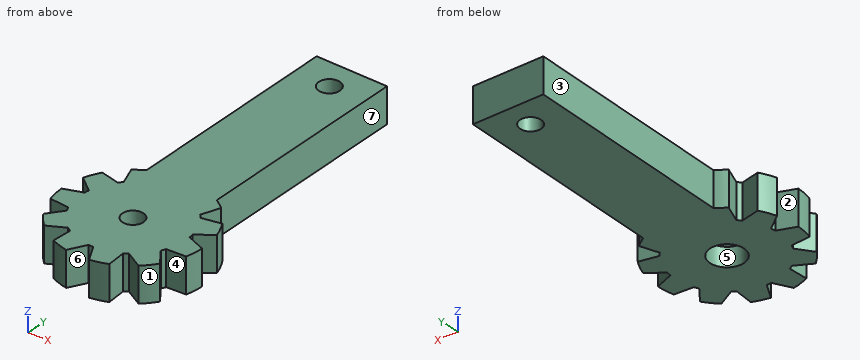
from build123d import *

# Parameters (mm, degrees)
BOSS_EXTRUDE1_DEPTH = 5
SKETCH5_R           = 2.425
CUT_EXTRUDE2_DEPTH  = 2.7
SKETCH6_R           = 1.5
CUT_EXTRUDE3_DEPTH  = 12
SKETCH7_W           = 10
SKETCH7_H           = 35
BOSS_EXTRUDE3_DEPTH = 5
SKETCH8_R           = 1.5
CUT_EXTRUDE4_DEPTH  = 12


with BuildPart() as part:
    # Sketch1 → Boss-Extrude1 (new body)
    with BuildSketch(Plane.XY):
        with BuildLine():
            Line((-1.212917817, 9.926168967), (-1.792316692, 7.28269187))
            ThreePointArc((-1.792316692, 7.28269187), (-2.112994176, 7.196197302), (-2.429527737, 7.095589826))
            Line((-2.429527737, 7.095589826), (-4.346120706, 9.006177592))
            ThreePointArc((-4.346120706, 9.006177592), (-5.406408175, 8.412535328), (-6.386863504, 7.694671831))
            Line((-6.386863504, 7.694671831), (-5.445113235, 5.157590703))
            ThreePointArc((-5.445113235, 5.157590703), (-5.668121808, 4.911455505), (-5.880014276, 4.655688147))
            Line((-5.880014276, 4.655688147), (-8.525296613, 5.226788465))
            ThreePointArc((-8.525296613, 5.226788465), (-9.096319954, 4.15415013), (-9.533025155, 3.020170756))
            Line((-9.533025155, 3.020170756), (-7.369124799, 1.394990929))
            ThreePointArc((-7.369124799, 1.394990929), (-7.423660814, 1.067361287), (-7.463637828, 0.737638377))
            Line((-7.463637828, 0.737638377), (-9.997751083, -0.212069068))
            ThreePointArc((-9.997751083, -0.212069068), (-9.898214419, -1.423148383), (-9.652518677, -2.613213194))
            Line((-9.652518677, -2.613213194), (-6.953491308, -2.810508608))
            ThreePointArc((-6.953491308, -2.810508608), (-6.822239965, -3.115612598), (-6.677609105, -3.414606366))
            Line((-6.677609105, -3.414606366), (-8.295990224, -5.583596171))
            ThreePointArc((-8.295990224, -5.583596171), (-7.557495744, -6.548607339), (-6.70740572, -7.416920419))
            Line((-6.70740572, -7.416920419), (-4.330173457, -6.12369152))
            ThreePointArc((-4.330173457, -6.12369152), (-4.054806131, -6.309401496), (-3.771486674, -6.482737714))
            Line((-3.771486674, -6.482737714), (-3.960311086, -9.182370941))
            ThreePointArc((-3.960311086, -9.182370941), (-2.817325568, -9.594929736), (-1.63273884, -9.865807817))
            Line((-1.63273884, -9.865807817), (-0.332056129, -7.492645643))
            ThreePointArc((-0.332056129, -7.492645643), (0, -7.5), (0.332056129, -7.492645643))
            Line((0.332056129, -7.492645643), (1.63273884, -9.865807817))
            ThreePointArc((1.63273884, -9.865807817), (2.817325568, -9.594929736), (3.960311086, -9.182370941))
            Line((3.960311086, -9.182370941), (3.771486674, -6.482737714))
            ThreePointArc((3.771486674, -6.482737714), (4.054806131, -6.309401496), (4.330173457, -6.12369152))
            Line((4.330173457, -6.12369152), (6.70740572, -7.416920419))
            ThreePointArc((6.70740572, -7.416920419), (7.557495744, -6.548607339), (8.295990224, -5.583596171))
            Line((8.295990224, -5.583596171), (6.677609105, -3.414606366))
            ThreePointArc((6.677609105, -3.414606366), (6.822239965, -3.115612598), (6.953491308, -2.810508608))
            Line((6.953491308, -2.810508608), (9.652518677, -2.613213194))
            ThreePointArc((9.652518677, -2.613213194), (9.898214419, -1.423148383), (9.997751083, -0.212069068))
            Line((9.997751083, -0.212069068), (7.463637828, 0.737638377))
            ThreePointArc((7.463637828, 0.737638377), (7.423660814, 1.067361287), (7.369124799, 1.394990929))
            Line((7.369124799, 1.394990929), (9.533025155, 3.020170756))
            ThreePointArc((9.533025155, 3.020170756), (9.096319954, 4.15415013), (8.525296613, 5.226788465))
            Line((8.525296613, 5.226788465), (5.880014276, 4.655688147))
            ThreePointArc((5.880014276, 4.655688147), (5.668121808, 4.911455505), (5.445113235, 5.157590703))
            Line((5.445113235, 5.157590703), (6.386863504, 7.694671831))
            ThreePointArc((6.386863504, 7.694671831), (5.406408175, 8.412535328), (4.346120706, 9.006177592))
            Line((4.346120706, 9.006177592), (2.429527737, 7.095589826))
            ThreePointArc((2.429527737, 7.095589826), (2.112994176, 7.196197302), (1.792316692, 7.28269187))
            Line((1.792316692, 7.28269187), (1.212917817, 9.926168967))
            ThreePointArc((1.212917817, 9.926168967), (0, 10), (-1.212917817, 9.926168967))
        make_face()
    extrude(amount=BOSS_EXTRUDE1_DEPTH)

    # Sketch5 → Cut-Extrude2 (cut)
    with BuildSketch(Plane(origin=(0, 0, 0), x_dir=(-1, 0, 0), z_dir=(0, 0, -1))):
        Circle(SKETCH5_R)
    extrude(amount=-CUT_EXTRUDE2_DEPTH, mode=Mode.SUBTRACT)

    # Sketch6 → Cut-Extrude3 (cut)
    with BuildSketch(Plane(origin=(0, 0, 2.7), x_dir=(-1, 0, 0), z_dir=(0, 0, -1))):
        Circle(SKETCH6_R)
    extrude(amount=-CUT_EXTRUDE3_DEPTH, mode=Mode.SUBTRACT)

    # Sketch7 → Boss-Extrude3 (add)
    with BuildSketch(Plane(origin=(0, 0, 0), x_dir=(-1, 0, 0), z_dir=(0, 0, -1))):
        with Locations((0, 21.5)):
            Rectangle(SKETCH7_W, SKETCH7_H)
    extrude(amount=-BOSS_EXTRUDE3_DEPTH)

    # Sketch8 → Cut-Extrude4 (cut)
    with BuildSketch(Plane(origin=(0, 0, 0), x_dir=(-1, 0, 0), z_dir=(0, 0, -1))):
        with Locations((0, 35)):
            Circle(SKETCH8_R)
    extrude(amount=-CUT_EXTRUDE4_DEPTH, mode=Mode.SUBTRACT)


solid = part.part
Build history of the part. All positions in model axes, mm. Face numbers are marked on the shaded views. A direction names the side the tool comes from. Give positions to 0.01 mm unless a question says otherwise; leave off trailing zeros. Order: outer loops, then holes, each group sorted by start corner. A loop starts at its lowest first (then second) coordinate and runs counter-clockwise, first axis right, second up. Notation, with made-up numbers: M 28,-5 L 83,-5 A30 cw 83,24 Z; hole C -30.5,49 d3. An arc over 180 degrees is marked long. Use one line per item in the form item = value.
1) Saw through at C-C (y = 18.5). Give the cut face in (x, z).
Calculated:
outline = M -5,0 L 5,0 L 5,5 L -5,5 Z
2) Two-plate mould, pull along Y, no slides. Class the marked faces 1, 2 and 3: released by +Y, released by -Y, zero draft, split by the parting line, or undercut.
Calculated:
face_1 = released by -Y
face_2 = undercut
face_3 = zero draft
3) Saw through at A-A (y = 35). Give the cut face in (x, z).
Calculated:
outline = M -5,0 L -1.5,0 L -1.5,5 L -5,5 Z; M 1.5,0 L 5,0 L 5,5 L 1.5,5 Z
4) Probe probe 1 along Y at (x, z) = (0, 3.5); probe 2 along Y at (x, z) = (0, 1.15) (3 decimals); probe 3 along X at (y, z) = (19.5, 4.8). List the from-to ranges inside material, lowest first.
Calculated:
probe_1 = -7.5 to -1.5, 1.5 to 33.5, 36.5 to 39
probe_2 = -7.5 to -2.425, 2.425 to 33.5, 36.5 to 39
probe_3 = -5 to 5
5) Drop flat-ended pins along their axis: pin 1 (4 mm diameter, centred on x = 0, y = 0, fed in from -Z); pin 2 (1 mm diameter, centred on y = 3.5, z = 2.5, fed in from +X); pin 3 (3 mm diameter, centred on x = -7.5, z = 1, fed in from +Y). Give the stop position or say it passes through.
Calculated:
pin_1 = 2.7
pin_2 = 9.53
pin_3 = 8
6) Tool access for the marked faces 4, 5, 6 and 7: list every direction of +Z, -Z, +X, -X, +Y, -Y with a clear straight run to the whole face (end or side of a thin tool).
Calculated:
face_4 = +Z, -Z, +X
face_5 = -Z
face_6 = +Z, -Z, -Y
face_7 = +Z, -Z, +X, +Y
7) Saw through at B-B (z = 1.45). State how many separate pieces and enclosed holes the cut face has, plus the area to 3 significant figures.
Calculated:
separate_pieces = 1
enclosed_holes = 2
area = 538 mm2
8) Saw through at D-D (y = -5). Give the cut face in (x, z).
Calculated:
outline = M -7.86,0 L 7.86,0 L 7.86,5 L -7.86,5 Z
